Source: CAD feature listing. Evaluate the final solid. Frame: model axes, mm. A direction names the side the tool comes from. Give positions to 0.01 mm unless a question says otherwise; leave off trailing zeros. Order: outer loops, then holes, each group sorted by start corner. A loop starts at its lowest first (then second) coordinate and runs counter-clockwise, first axis right, second up.
from build123d import *

# Parameters (mm, degrees)
F0_R     = 55.407722
F1_DEPTH = 44.196
F2_R     = 37.543848
F3_DEPTH = 71.882
F4_R     = 5.08


with BuildPart() as f1:
    # F0 (on Front) → F1 (new body)
    with BuildSketch(Plane.XZ):
        Circle(F0_R)
    extrude(amount=F1_DEPTH)

    # F2 (on Front) → F3 (join)
    with BuildSketch(Plane.XZ):
        Circle(F2_R)
    extrude(amount=F3_DEPTH)

    # F4
    f4_edges = [f1.edges().sort_by_distance(p)[0] for p in [
        (-37.543848, -71.882, 0),
        (-55.407722, -44.196, 0),
    ]]
    fillet(f4_edges, radius=F4_R)


solid = f1.part
1) Section query A-A on x = 0. Output: boundary loops of the cut face in (y, z), and give its area (3 significant figures).
Checks:
outline: (-71.88, -32.46) arc R5.08 ccw to (-66.8, -37.54) - (-44.2, -37.54) - (-44.2, -50.33) arc R5.08 ccw to (-39.12, -55.41) - (0, -55.41) - (0, 55.41) - (-39.12, 55.41) arc R5.08 ccw to (-44.2, 50.33) - (-44.2, 37.54) - (-66.8, 37.54) arc R5.08 ccw to (-71.88, 32.46) - close
area: 6,950 mm2
2) First-contact query: pin 1 Ø10 at (x, y) = (13.5, -26) entering from +Z; pin 2 Ø10 at (x, y) = (39, -14) entering from -Z; pin 3 Ø6 at (y, z) = (-15.5, -23) entering from -X. Flat tips, straight axial feed; report the tip coordinate or a pass-through.
Checks:
pin 1: stops at z = 54.75
pin 2: stops at z = -43.75
pin 3: stops at x = -51.67
3) Reachability of faces 1 (the face through (-38, -44.196, -3)), 2 (the face through (0, -71.882, 0)) from +Z, -Z, +X, -X, +Y, -Y: full face, straight path, thin tool, end or side. Return the list, or none.
Checks:
face 1: -Y
face 2: +Z, -Z, +X, -X, -Y
4) Section query D-D on y = -35.5. Output: boundary loops of the cut face in (x, z), and give its area (3 significant figures).
Checks:
outline: circle Ø110.82 at (0, 0)
area: 9,640 mm2
5) Section query B-B on z = 0. Output: boundary loops of the cut face in (x, y).
Checks:
outline: (-55.41, -39.12) arc R5.08 ccw to (-50.33, -44.2) - (-37.54, -44.2) - (-37.54, -66.8) arc R5.08 ccw to (-32.46, -71.88) - (32.46, -71.88) arc R5.08 ccw to (37.54, -66.8) - (37.54, -44.2) - (50.33, -44.2) arc R5.08 ccw to (55.41, -39.12) - (55.41, 0) - (-55.41, 0) - close
6) Ray query, L1, parallel to Y at x = 21, z = -32; L2, parallel to Z at x = -1.5, y = -22; L3, parallel to X at y = -35, z = 46.5. Return the intervals inside material, ascending.
Checks:
L1: y = -44.2 to 0
L2: z = -55.39 to 55.39
L3: x = -30.13 to 30.13
7) Section query C-C on y = -59.5. Output: boundary loops of the cut face in (x, z), and give its area (3 significant figures).
Checks:
outline: circle Ø75.09 at (0, 0)
area: 4,430 mm2
